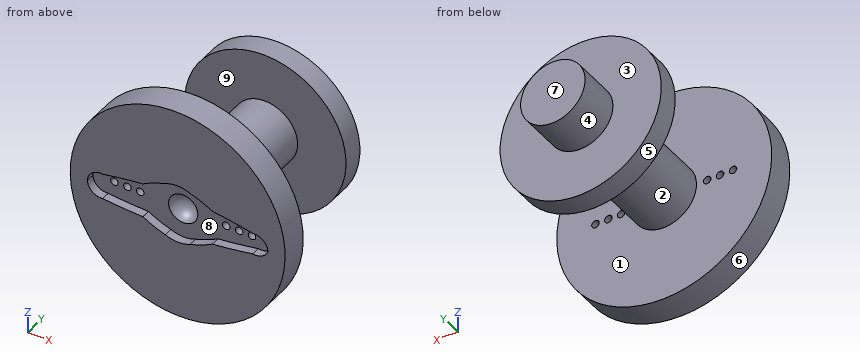
from build123d import *

# Parameters (mm, degrees)
SKETCH1_R             = 25
BOSS_EXTRUDE1_DEPTH   = 6.5
HORN_HOLE_DEPTH       = 2
SCREW_HOLES_REACH     = 37.641
SKETCH9_R             = 0.875
SKETCH11_R            = 7.5
BOSS_EXTRUDE2_DEPTH   = 25
SKETCH12_R            = 18.75
BOSS_EXTRUDE3_DEPTH   = 5
SCREW_HEAD_HOLE_ANGLE = 180
BOSS_EXTRUDE4_START   = 30
SKETCH11_2_R          = 7.5
BOSS_EXTRUDE4_DEPTH   = 10


with BuildPart() as part:
    # Sketch1 → Boss-Extrude1 (new body)
    with BuildSketch(Plane(origin=(0, 0, 0), x_dir=(1, 0, 0), z_dir=(0, 1, 0))):
        with Locations(Location((0, 0, 0), (0, 0, 90))):
            Circle(SKETCH1_R)
    extrude(amount=BOSS_EXTRUDE1_DEPTH)

    # Sketch8 → Horn Hole (cut)
    with BuildSketch(Plane.XZ):
        with BuildLine():
            ThreePointArc((2.867832451, 6.276606431), (5.55485913, 5.311303559), (8.103473198, 4.024257195))
            ThreePointArc((8.103473198, 4.024257195), (12.790122891, 3.37163327), (17.445502266, 2.524257195))
            ThreePointArc((17.445502266, 2.524257195), (19.894779582, 1.820498395), (21, -0.475742805))
            ThreePointArc((21, -0.475742805), (19.60737188, -2.167378066), (17.445502266, -2.524257195))
            ThreePointArc((17.445502266, -2.524257195), (12.790122891, -3.37163327), (8.103473198, -4.024257195))
            ThreePointArc((8.103473198, -4.024257195), (5.55485913, -5.311303559), (2.867832451, -6.276606431))
            ThreePointArc((2.867832451, -6.276606431), (0, -6.900742805), (-2.867832451, -6.276606431))
            ThreePointArc((-2.867832451, -6.276606431), (-5.55485913, -5.311303559), (-8.103473198, -4.024257195))
            ThreePointArc((-8.103473198, -4.024257195), (-12.780142502, -3.846309279), (-17.445502266, -3.475742805))
            ThreePointArc((-17.445502266, -3.475742805), (-19.894779582, -2.771984005), (-21, -0.475742805))
            ThreePointArc((-21, -0.475742805), (-19.894779582, 1.820498395), (-17.445502266, 2.524257195))
            ThreePointArc((-17.445502266, 2.524257195), (-12.790122891, 3.37163327), (-8.103473198, 4.024257195))
            ThreePointArc((-8.103473198, 4.024257195), (-5.55485913, 5.311303559), (-2.867832451, 6.276606431))
            ThreePointArc((-2.867832451, 6.276606431), (0, 6.900742805), (2.867832451, 6.276606431))
        make_face()
    extrude(amount=-HORN_HOLE_DEPTH, mode=Mode.SUBTRACT)

    # Sketch9 → Screw Holes (cut, up to next)
    with BuildSketch(Plane.XZ.offset(-2), mode=Mode.PRIVATE) as screw_holes_sk1:
        with Locations(Location((10, 0, 0), (0, 0, 270))):
            Circle(SKETCH9_R)
    screw_holes_tool1 = extrude(screw_holes_sk1.sketch, amount=-SCREW_HOLES_REACH, mode=Mode.PRIVATE) & part.part
    # Sketch9 → Screw Holes (cut, up to next)
    with BuildSketch(Plane.XZ.offset(-2), mode=Mode.PRIVATE) as screw_holes_sk2:
        with Locations(Location((13, 0, 0), (0, 0, 270))):
            Circle(SKETCH9_R)
    screw_holes_tool2 = extrude(screw_holes_sk2.sketch, amount=-SCREW_HOLES_REACH, mode=Mode.PRIVATE) & part.part
    # Sketch9 → Screw Holes (cut, up to next)
    with BuildSketch(Plane.XZ.offset(-2), mode=Mode.PRIVATE) as screw_holes_sk3:
        with Locations(Location((16, 0, 0), (0, 0, 270))):
            Circle(SKETCH9_R)
    screw_holes_tool3 = extrude(screw_holes_sk3.sketch, amount=-SCREW_HOLES_REACH, mode=Mode.PRIVATE) & part.part
    # Sketch9 → Screw Holes (cut, up to next)
    with BuildSketch(Plane.XZ.offset(-2), mode=Mode.PRIVATE) as screw_holes_sk4:
        with Locations(Location((-10, 0, 0), (0, 0, 90))):
            Circle(SKETCH9_R)
    screw_holes_tool4 = extrude(screw_holes_sk4.sketch, amount=-SCREW_HOLES_REACH, mode=Mode.PRIVATE) & part.part
    # Sketch9 → Screw Holes (cut, up to next)
    with BuildSketch(Plane.XZ.offset(-2), mode=Mode.PRIVATE) as screw_holes_sk5:
        with Locations(Location((-13, 0, 0), (0, 0, 90))):
            Circle(SKETCH9_R)
    screw_holes_tool5 = extrude(screw_holes_sk5.sketch, amount=-SCREW_HOLES_REACH, mode=Mode.PRIVATE) & part.part
    # Sketch9 → Screw Holes (cut, up to next)
    with BuildSketch(Plane.XZ.offset(-2), mode=Mode.PRIVATE) as screw_holes_sk6:
        with Locations(Location((-16, 0, 0), (0, 0, 90))):
            Circle(SKETCH9_R)
    screw_holes_tool6 = extrude(screw_holes_sk6.sketch, amount=-SCREW_HOLES_REACH, mode=Mode.PRIVATE) & part.part
    add(screw_holes_tool1.solids().sort_by_distance((10, 2, 0))[0], mode=Mode.SUBTRACT)
    add(screw_holes_tool2.solids().sort_by_distance((13, 2, 0))[0], mode=Mode.SUBTRACT)
    add(screw_holes_tool3.solids().sort_by_distance((16, 2, 0))[0], mode=Mode.SUBTRACT)
    add(screw_holes_tool4.solids().sort_by_distance((-10, 2, 0))[0], mode=Mode.SUBTRACT)
    add(screw_holes_tool5.solids().sort_by_distance((-13, 2, 0))[0], mode=Mode.SUBTRACT)
    add(screw_holes_tool6.solids().sort_by_distance((-16, 2, 0))[0], mode=Mode.SUBTRACT)

    # Sketch11 → Boss-Extrude2 (add)
    with BuildSketch(Plane(origin=(0, 6.5, 0), x_dir=(1, 0, 0), z_dir=(0, 1, 0))):
        with Locations(Location((0, 0, 0), (0, 0, 270))):
            Circle(SKETCH11_R)
    extrude(amount=BOSS_EXTRUDE2_DEPTH)

    # Sketch12 → Boss-Extrude3 (add)
    with BuildSketch(Plane(origin=(0, 31.5, 0), x_dir=(1, 0, 0), z_dir=(0, 1, 0))):
        with Locations(Location((0, 0, 0), (0, 0, 270))):
            Circle(SKETCH12_R)
    extrude(amount=BOSS_EXTRUDE3_DEPTH)

    # Sketch13 → Screw Head Hole (revolve, cut)
    with BuildSketch(Plane.XZ.offset(-2)):
        with BuildLine():
            Line((3.4, 0), (-3.4, 0))
            ThreePointArc((-3.4, 0), (0, -3.4), (3.4, 0))
        make_face()
    revolve(axis=Axis((3.4, 2, 0), (1, 0, 0)), revolution_arc=SCREW_HEAD_HOLE_ANGLE, mode=Mode.SUBTRACT)

    # Sketch11<2> → Boss-Extrude4 (add)
    with BuildSketch(Plane(origin=(0, 6.5, 0), x_dir=(1, 0, 0), z_dir=(0, 1, 0)).offset(BOSS_EXTRUDE4_START)):
        with Locations(Location((0, 0, 0), (0, 0, 270))):
            Circle(SKETCH11_2_R)
    extrude(amount=BOSS_EXTRUDE4_DEPTH)


solid = part.part
Geometry check sheet. Reference: the model listing, model coordinates, mm. Face numbers are marked on the shaded views. A direction names the side the tool comes from. Round coordinates to 2 decimals unless told otherwise and drop trailing zeros. Order: outer loops, then holes, each group sorted by start corner. A loop starts at its lowest first (then second) coordinate and runs counter-clockwise, first axis right, second up. Notation, with made-up numbers: M 14,17.25 L 54,17.25 A11 cw 54,37.25 Z; hole C -4.5,83.5 d10. An arc over 180 degrees is marked long. Write each question's results on one line, items separated by ' | '. Start each with the question number.
1. Draft check along Y on the marked faces 1, 2, 3 and 4. Enter one of: pulls with the +Y half, pulls with the -Y half, needs draft (parallel to the pull), parting line crosses it, or undercut.
2. Go/stop test with flat-tipped pins: P1, Ø1.6, axis at x = 13, z = 0, coming from the -Y side; P2, Ø2, axis at x = -16, z = 0, coming from the -Y side; P3, Ø1.1, axis at x = 16, z = 0, coming from the +Y side. Record where each tip stops, or that it passes through.
3. Cross-section at B-B on z = 11. Record the boundary of the cut face in (x, y).
4. Material ranges on L1, parallel to Y at x = 13, z = 5.5; L2, parallel to Y at x = -12, z = 0; L3, parallel to Z at x = -0.5, y = 32.5, recorded low to high. Write a range as from..to.
5. Set-up check for the marked faces 5, 6, 7, 8 and 9: record each of +Z, -Z, +X, -X, +Y, -Y from which the full face is reachable in a straight line by a thin tool's end or side.
6. Cross-section at D-D on x = 13. Record the boundary of the cut face in (y, z) (3 decimals), plus the area to 3 significant figures.
7. Cross-section at A-A on x = -13. Record the boundary of the cut face in (y, z) (3 decimals), plus the area to 3 significant figures.
8. Cross-section at C-C on z = -20. Record the boundary of the cut face in (x, y), plus the area to 3 significant figures.
Resolved:
1) face 1: undercut | face 2: undercut | face 3: pulls with the +Y half | face 4: needs draft
2) P1: y = 31.5 | P2: y = 2 | P3: y = 36.5
3) outline: M -22.45,0 L 22.45,0 L 22.45,6.5 L -22.45,6.5 Z; M -15.18,31.5 L 15.18,31.5 L 15.18,36.5 L -15.18,36.5 Z
4) L1: 0..6.5, 31.5..36.5 | L2: 2..6.5, 31.5..36.5 | L3: -18.74..18.74
5) face 5: +Y | face 6: +Y, -Y | face 7: +Z, -Z, +X, -X, +Y | face 8: -Y | face 9: none
6) outline: M 0,-21.354 L 6.5,-21.354 L 6.5,-0.875 L 2,-0.875 L 2,-3.338 L 0,-3.338 Z; M 0,3.338 L 2,3.338 L 2,0.875 L 6.5,0.875 L 6.5,21.354 L 0,21.354 Z; M 31.5,-13.512 L 36.5,-13.512 L 36.5,13.512 L 31.5,13.512 Z | area: 391 mm2
7) outline: M 0,-21.354 L 6.5,-21.354 L 6.5,-0.875 L 2,-0.875 L 2,-3.833 L 0,-3.833 Z; M 0,3.338 L 2,3.338 L 2,0.875 L 6.5,0.875 L 6.5,21.354 L 0,21.354 Z; M 31.5,-13.512 L 36.5,-13.512 L 36.5,13.512 L 31.5,13.512 Z | area: 391 mm2
8) outline: M -15,0 L 15,0 L 15,6.5 L -15,6.5 Z | area: 195 mm2
